from build123d import *

# Parameters (mm, degrees)
BOSS_EXTRUDE1_DEPTH = 38.1
BOSS_EXTRUDE2_START = 10.16
SKETCH2_R           = 3.175
BOSS_EXTRUDE2_DEPTH = 10.16
CHAMFER1_SIZE       = 15.24


with BuildPart() as part:
    # Sketch1 → Boss-Extrude1 (new body)
    with BuildSketch(Plane(origin=(0, 0, 0), x_dir=(1, 0, 0), z_dir=(0, 1, 0))):
        with BuildLine():
            Line((-3.175, 0), (-3.175, 120.65))
            ThreePointArc((-3.175, 120.65), (0, 123.825), (3.175, 120.65))
            Line((3.175, 120.65), (3.175, 3.175))
            Line((3.175, 3.175), (66.675, 3.175))
            Line((66.675, 3.175), (66.675, 120.65))
            ThreePointArc((66.675, 120.65), (69.85, 123.825), (73.025, 120.65))
            Line((73.025, 120.65), (73.025, 0))
            ThreePointArc((73.025, 0), (72.09506403, -2.24506403), (69.85, -3.175))
            Line((69.85, -3.175), (0, -3.175))
            ThreePointArc((0, -3.175), (-2.24506403, -2.24506403), (-3.175, 0))
        make_face()
    extrude(amount=BOSS_EXTRUDE1_DEPTH)

    # Sketch2 → Boss-Extrude2 (add)
    with BuildSketch(Plane(origin=(0, 0, 0), x_dir=(-1, 0, 0), z_dir=(0, -1, 0)).offset(BOSS_EXTRUDE2_START)):
        with Locations(Location((-69.85, 120.65, 0), (0, 0, 90))):
            Circle(SKETCH2_R)
        with Locations(Location((0, 120.65, 0), (0, 0, 90))):
            Circle(SKETCH2_R)
        with Locations(Location((0, 0, 0), (0, 0, 90))):
            Circle(SKETCH2_R)
        with Locations(Location((-69.85, 0, 0), (0, 0, 90))):
            Circle(SKETCH2_R)
    extrude(amount=-BOSS_EXTRUDE2_DEPTH)

    # Chamfer1
    chamfer1_edges = [part.edges().sort_by_distance(p)[0] for p in [
        (3.175, 19.05, -3.175),
        (66.675, 19.05, -3.175),
    ]]
    chamfer(chamfer1_edges, length=CHAMFER1_SIZE)


solid = part.part
Geometry: final body of the model. Coordinates: model frame, mm. A direction names the side the tool comes from. Give positions to 0.01 mm unless a question says otherwise; leave off trailing zeros. Order: outer loops, then holes, each group sorted by start corner. A loop starts at its lowest first (then second) coordinate and runs counter-clockwise, first axis right, second up. Notation, with made-up numbers: (-34, 25) -> (-23, 25) arc R26 ccw to (-23, 59) -> close; hole circle Ø2 at (81.25, 76.5). An arc over 180 degrees is marked (long way). Write each question's results on one line, items separated by ' | '.
1) First-contact query: pin 1 Ø5 at (x, z) = (9.5, -14.5) entering from -Y. Flat tip, straight axial feed; report the tip coordinate or a pass-through.
Geometry says:
pin 1: stops at y = 0
2) Cut plane D-D (y = 11). Output: boundary loops of the cut face in (x, z) (3 decimals), and give its area (3 significant figures).
Geometry says:
outline: (-3.175, -120.65) arc R3.175 ccw to (3.175, -120.65) -> (3.175, -18.415) -> (18.415, -3.175) -> (51.435, -3.175) -> (66.675, -18.415) -> (66.675, -120.65) arc R3.175 ccw to (73.025, -120.65) -> (73.025, 0) arc R3.175 ccw to (69.85, 3.175) -> (0, 3.175) arc R3.175 ccw to (-3.175, 0) -> close | area: 2,240 mm²
3) Set-up query: faces 4 (the face through (69, 38.1, -47)), 5 (the face through (58.95, 18.78, -10.69)). Return all of +Z, -Z, +X, -X, +Y, -Y with unobstructed straight access to the full face (end or side cutting, diameter ignored); none if empty.
Geometry says:
face 4: +Z, -Z, +X, -X, +Y | face 5: -Z, +Y, -Y
4) Line query: line 1 along X through (y, z) = (8, -49.5) (3 decimals); line 2 along Z through (x, y) = (42.5, 30.5) (3 decimals); line 3 along Y through (x, z) = (7, -4). Output: solid intervals per line, ascending.
Geometry says:
line 1: x = -3.175 to 3.175, 66.675 to 73.025 | line 2: z = -3.175 to 3.175 | line 3: y = 0 to 38.1
5) Draft query along Z for faces 1 (the face through (35, 19, -3.175)), 2 (the face through (35, 19, 3.175)), 3 (the face through (69, 0, -45)). Return one class per face: released by +Z, released by -Z, zero draft, split by the parting line, or undercut.
Geometry says:
face 1: released by -Z | face 2: released by +Z | face 3: undercut
6) Cut plane B-B (y = -3.5). Output: boundary loops of the cut face in (x, z) (3 decimals), and give its area (3 significant figures).
Geometry says:
outline: circle Ø6.35 at (0, -120.65); circle Ø6.35 at (0, 0); circle Ø6.35 at (69.85, -120.65); circle Ø6.35 at (69.85, 0) | area: 127 mm²
7) Cut plane A-A (z = -15.5). Output: boundary loops of the cut face in (x, y) (3 decimals), and give its area (3 significant figures).
Geometry says:
outline: (-3.175, 0) -> (6.09, 0) -> (6.09, 38.1) -> (-3.175, 38.1) -> close; (63.76, 0) -> (73.025, 0) -> (73.025, 38.1) -> (63.76, 38.1) -> close | area: 706 mm²
8) Cut plane C-C (z = -39.5). Output: boundary loops of the cut face in (x, y) (3 decimals).
Geometry says:
outline: (-3.175, 0) -> (3.175, 0) -> (3.175, 38.1) -> (-3.175, 38.1) -> close; (66.675, 0) -> (73.025, 0) -> (73.025, 38.1) -> (66.675, 38.1) -> close
